Design review of the part built by this model. Coordinates are the model's own, in mm. A direction names the side the tool comes from. Coordinates: 2 decimals unless noted, no trailing zeros. Loops run counter-clockwise (first coordinate to the right, second up) from the corner with the lowest first, then second, coordinate; pieces in that order, holes last. Notation, with made-up numbers: (38.5, -9.5) -> (84.5, -9.5) arc R18 ccw to (84.5, 10.5) -> close; hole circle Ø10 at (-4.75, 40). An arc over 180 degrees is marked (long way). Answer in a Markdown table with one row per item.
```python
from build123d import *

# Parameters (mm, degrees)
SKETCH1_W               = 20
SKETCH1_H               = 174
MIDLINE_SUPPORT_DEPTH   = 6
SKETCH7_R               = 1.75
FRONT_SCREW_HOLES_DEPTH = 10


with BuildPart() as part:
    # Sketch1 → Midline Support (new body)
    with BuildSketch(Plane(origin=(0, 0, 0), x_dir=(1, 0, 0), z_dir=(0, 1, 0))):
        Rectangle(SKETCH1_W, SKETCH1_H)
    extrude(amount=MIDLINE_SUPPORT_DEPTH)

    # Sketch7 → Front Screw Holes (cut)
    with BuildSketch(Plane.XY.offset(87)):
        with Locations((-5, 3)):
            Circle(SKETCH7_R)
        with Locations(Location((5, 3, 0), (0, 0, 180))):
            Circle(SKETCH7_R)
    front_screw_holes = extrude(amount=-FRONT_SCREW_HOLES_DEPTH, mode=Mode.SUBTRACT)

    # Rear Screw Holes: Front Screw Holes across plane
    add(front_screw_holes.mirror(Plane.XY), mode=Mode.SUBTRACT)


solid = part.part
```
(1) Tool access review of faces 5 (the flat face through (0, 3, 87)), 6 (the flat face through (5, 3, 77)), 7 (the flat face through (5, 3, -77)): name each direction out of +Z, -Z, +X, -X, +Y, -Y from which nothing blocks a thin tool from reaching the whole face with its end or side.
Evaluation:
| item | result |
|---|---|
| face 5 | +Z, +X, -X, +Y, -Y |
| face 6 | +Z |
| face 7 | -Z |
(2) Draft analysis for pull direction X (two halves, no side actions). For faces 1 (the flat face through (-10, 3, 1)), 2 (the flat face through (10, 3, 1)), 3 (the flat face through (0, 3, -87)), 4 (the flat face through (-5, 3, 77)), state which applies: pulls with the +X half, pulls with the -X half, needs draft (parallel to the pull), parting line crosses it, or undercut.
Evaluation:
| item | result |
|---|---|
| face 1 | pulls with the -X half |
| face 2 | pulls with the +X half |
| face 3 | needs draft |
| face 4 | undercut |
(3) Take a section at A-A on x = 5. Give the boundary of the cut face in (y, z), and give its area (3 significant figures).
Evaluation:
| item | result |
|---|---|
| outline | (0, -87) -> (1.25, -87) -> (1.25, -77) -> (4.75, -77) -> (4.75, -87) -> (6, -87) -> (6, 87) -> (4.75, 87) -> (4.75, 77) -> (1.25, 77) -> (1.25, 87) -> (0, 87) -> close |
| area | 974 mm² |
(4) To check wall thickness, follow probe 1 along Y at (x, z) = (5, -84); probe 2 along Z at (x, y) = (-5.25, 2.35). State the ranges of each line that lie inside material, in increasing order.
Evaluation:
| item | result |
|---|---|
| probe 1 | y = 0 to 1.25, 4.75 to 6 |
| probe 2 | z = -77 to 77 |
(5) For pin 1 (2 mm diameter, centred on x = 5, y = 3, fed in from +Z); pin 2 (1.8 mm diameter, centred on x = 5, y = 3.5, fed in from -Z), all flat-tipped, find the tip position at first contact; note any pin that passes through.
Evaluation:
| item | result |
|---|---|
| pin 1 | stops at z = 77 |
| pin 2 | stops at z = -77 |
